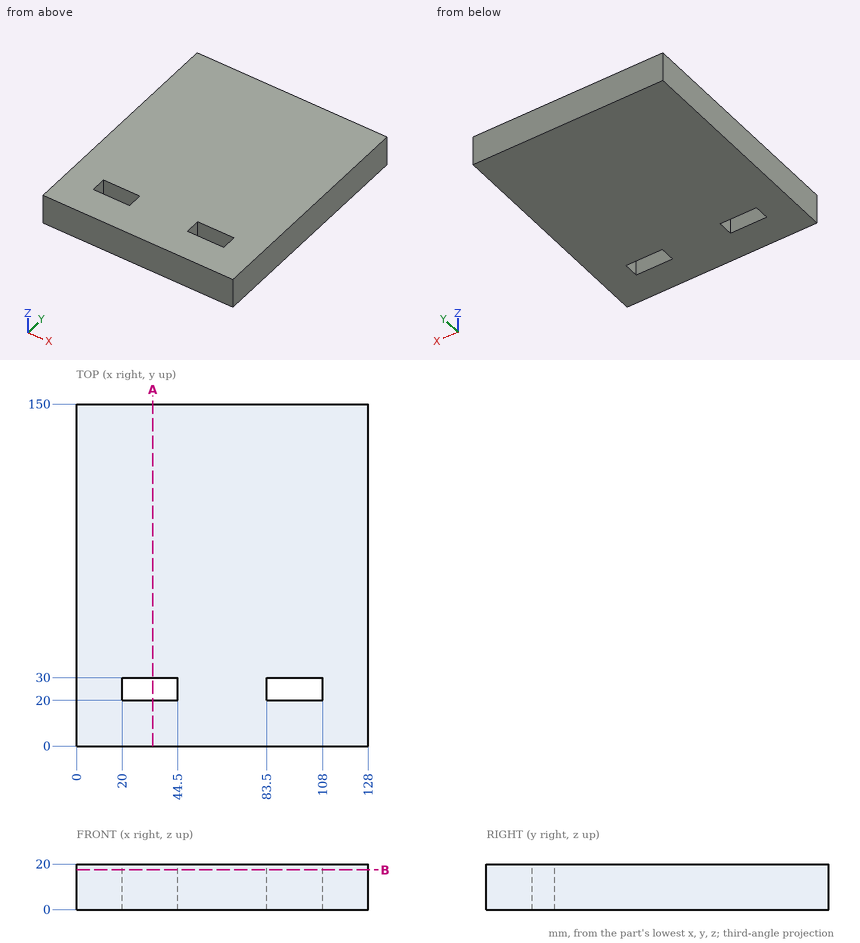
Input: dimensioned drawing with shaded views. Units: mm. Origin: part minimum x, y, z. Round coordinates to 2 decimals unless told otherwise and drop trailing zeros. Order: outer loops, then holes, each group sorted by start corner. A loop starts at its lowest first (then second) coordinate and runs counter-clockwise, first axis right, second up. Notation, with made-up numbers: (70.25, 36.25) - (86.25, 36.25) arc R25 ccw to (86.25, 62.25) - close; hole circle Ø10 at (81.25, 88.5). An arc over 180 degrees is marked (long way). Answer as a JSON object with one key per item and string values. Group by question number.
(1) Cut plane B-B (z = 17.5). Return loops of the section in (x, y).
(2) Pin query (flat end, axial travel): P1, Ø6, axis at x = 14.5, y = 113.5, coming from the -Z side. Return the tip coordinate at first contact, or that it passes through.
(3) Material intervals for probe 1 along X at (y, z) = (27, 9.75); probe 2 along Y at (x, z) = (26.5, 7), sorted ascending. Write a range as from..to.
(4) Cut plane A-A (x = 33.5). Return loops of the section in (y, z).
Here are the results:
{
 "1": {"outline": "(0, 0) - (128, 0) - (128, 150) - (0, 150) - close; hole (20, 20) - (44.5, 20) - (44.5, 30) - (20, 30) - close; hole (83.5, 20) - (108, 20) - (108, 30) - (83.5, 30) - close"},
 "2": {"P1": "stops at z = 0"},
 "3": {"probe 1": "x = 0..20, 44.5..83.5, 108..128", "probe 2": "y = 0..20, 30..150"},
 "4": {"outline": "(0, 0) - (20, 0) - (20, 20) - (0, 20) - close; (30, 0) - (150, 0) - (150, 20) - (30, 20) - close"}
}
